Source: CAD feature listing. Evaluate the final solid. Frame: model axes, mm. A direction names the side the tool comes from. Round coordinates to 2 decimals unless told otherwise and drop trailing zeros. Loops run counter-clockwise (first coordinate to the right, second up) from the corner with the lowest first, then second, coordinate; pieces in that order, holes last. Notation, with made-up numbers: (-25, 79) -> (24, 79) arc R28 cw to (24, 99) -> close; hole circle Ø2 at (55.5, 74). An arc over 180 degrees is marked (long way). Write item = value, one per line.
from build123d import *

# Parameters (mm, degrees)
EXTRUDE_1_DEPTH              = 7
HOLE_WIZARD_M3_2_D           = 3.2
HOLE_WIZARD_M3_2_DEPTH       = 7
HOLE_WIZARD_M3_2_CBORE_D     = 6.2
HOLE_WIZARD_M3_2_CBORE_DEPTH = 1.3
HOLE_WIZARD_M3_2_TIP         = 0.96137699
CUT_EXTRUDE_1_DEPTH          = 2
EXTRUDE_START                = -3.5
EXTRUDE_3_DEPTH              = 1.5
FILLET_1_R                   = 2
CHAMFER_1_SIZE               = 0.5
CHAMFER_1_SIZE2              = 0.866025404
FILLET_2_R                   = 1
CHAMFER_2_SIZE               = 0.5
DELETE_START                 = 2
DELETE_FACE_1_DEPTH          = 3
DELETE_FACE_2_DEPTH          = 3
FILLET_3_R                   = 3.5
CHAMFER_3_SIZE               = 0.3


with BuildPart() as part:
    # 草图1 → 凸台-拉伸1 (new body)
    with BuildSketch(Plane(origin=(0, 0, 0), x_dir=(1, 0, 0), z_dir=(0, 1, 0))):
        Polygon((12.5, -5.17766953), (12.5, 5.17766953), (5.17766953, 12.5), (-5.17766953, 12.5), (-12.5, 5.17766953), (-12.5, -5.17766953), (-5.17766953, -12.5), (5.17766953, -12.5), align=None)
    extrude(amount=EXTRUDE_1_DEPTH)

    # M3 六角圆柱头螺钉的柱形沉头孔2
    with Locations(Plane.XZ):
        with Locations((-5.25, 0), (0, 5.25), (5.25, 0), (0, -5.25)):
            CounterBoreHole(HOLE_WIZARD_M3_2_D / 2, HOLE_WIZARD_M3_2_CBORE_D / 2, HOLE_WIZARD_M3_2_CBORE_DEPTH, depth=HOLE_WIZARD_M3_2_DEPTH)
            with Locations((0, 0, -(HOLE_WIZARD_M3_2_DEPTH + HOLE_WIZARD_M3_2_TIP / 2))):  # 118° drill point
                Cone(0, HOLE_WIZARD_M3_2_D / 2, HOLE_WIZARD_M3_2_TIP, mode=Mode.SUBTRACT)

    # 草图7 → 切除-拉伸1 (cut)
    with BuildSketch(Plane(origin=(0, 7, 0), x_dir=(1, 0, 0), z_dir=(0, 1, 0))):
        with BuildLine():
            Line((-1, 2), (1, 2))
            ThreePointArc((1, 2), (3, 0), (1, -2))
            Line((1, -2), (-1, -2))
            ThreePointArc((-1, -2), (-3, 0), (-1, 2))
        make_face()
    extrude(amount=-CUT_EXTRUDE_1_DEPTH, mode=Mode.SUBTRACT)

    # 草图8 → 凸台-拉伸3 (add, symmetric)
    with BuildSketch(Plane(origin=(0, 7, 0), x_dir=(1, 0, 0), z_dir=(0, 1, 0)).offset(EXTRUDE_START)):
        Polygon((5.798989873, 14), (-5.798989873, 14), (-14, 5.798989873), (-14, -5.798989873), (-5.798989873, -14), (5.798989873, -14), (14, -5.798989873), (14, 5.798989873), align=None)
        Polygon((12.5, 5.17766953), (5.17766953, 12.5), (-5.17766953, 12.5), (-12.5, 5.17766953), (-12.5, -5.17766953), (-5.17766953, -12.5), (5.17766953, -12.5), (12.5, -5.17766953), align=None, mode=Mode.SUBTRACT)
    extrude(amount=EXTRUDE_3_DEPTH, both=True)

    # 圆角1
    fillet_1_edges = [part.edges().sort_by_distance(p)[0] for p in [
        (5.17766953, 6, 12.5),
        (-5.17766953, 6, 12.5),
        (-12.5, 6, 5.17766953),
        (-12.5, 6, -5.17766953),
        (-5.17766953, 6, -12.5),
        (5.17766953, 6, -12.5),
        (12.5, 6, -5.17766953),
        (12.5, 6, 5.17766953),
        (5.17766953, 1, 12.5),
        (-5.17766953, 1, 12.5),
        (-12.5, 1, 5.17766953),
        (-12.5, 1, -5.17766953),
        (-5.17766953, 1, -12.5),
        (5.17766953, 1, -12.5),
        (12.5, 1, -5.17766953),
        (12.5, 1, 5.17766953),
        (14, 3.5, -5.798989873),
        (5.798989873, 3.5, -14),
        (-5.798989873, 3.5, -14),
        (-14, 3.5, -5.798989873),
        (-14, 3.5, 5.798989873),
        (-5.798989873, 3.5, 14),
        (5.798989873, 3.5, 14),
        (14, 3.5, 5.798989873),
    ]]
    fillet(fillet_1_edges, radius=FILLET_1_R)

    # 倒角1
    chamfer_1_edges = [part.edges().sort_by_distance(p)[0] for p in [
        (-3, 7, 0),
        (0, 7, 2),
        (3, 7, 0),
        (0, 7, -2),
    ]]
    chamfer_1_side = [part.faces().sort_by_distance(p)[0] for p in [
        (12.146446609, 7, 0),
    ]]
    chamfer(chamfer_1_edges, length=CHAMFER_1_SIZE, length2=CHAMFER_1_SIZE2, reference=chamfer_1_side[0])

    # 圆角2
    fillet_2_edges = [part.edges().sort_by_distance(p)[0] for p in [
        (9.899494937, 2, -9.899494937),
        (9.899494937, 5, -9.899494937),
        (14, 2, 0),
        (9.899494937, 2, 9.899494937),
        (0, 2, 14),
        (-9.899494937, 2, 9.899494937),
        (-14, 2, 0),
        (-9.899494937, 2, -9.899494937),
        (0, 2, -14),
        (-13.847759065, 2, -5.735929613),
        (5.735929613, 2, -13.847759065),
        (-5.735929613, 2, -13.847759065),
        (-13.847759065, 2, 5.735929613),
        (-5.735929613, 2, 13.847759065),
        (5.735929613, 2, 13.847759065),
        (13.847759065, 2, 5.735929613),
        (13.847759065, 2, -5.735929613),
        (14, 5, 0),
        (0, 5, -14),
        (-9.899494937, 5, -9.899494937),
        (-14, 5, 0),
        (-9.899494937, 5, 9.899494937),
        (0, 5, 14),
        (9.899494937, 5, 9.899494937),
        (-13.847759065, 5, -5.735929613),
        (5.735929613, 5, -13.847759065),
        (-5.735929613, 5, -13.847759065),
        (-13.847759065, 5, 5.735929613),
        (-5.735929613, 5, 13.847759065),
        (5.735929613, 5, 13.847759065),
        (13.847759065, 5, 5.735929613),
        (13.847759065, 5, -5.735929613),
    ]]
    fillet(fillet_2_edges, radius=FILLET_2_R)

    # 倒角2
    chamfer_2_edges = [part.edges().sort_by_distance(p)[0] for p in [
        (12.5, 0, 0),
        (8.838834765, 0, 8.838834765),
        (0, 0, 12.5),
        (-8.838834765, 0, 8.838834765),
        (-12.5, 0, 0),
        (-8.838834765, 0, -8.838834765),
        (0, 0, -12.5),
        (8.838834765, 0, -8.838834765),
        (-12.347759065, 0, -5.11460927),
        (12.347759065, 0, -5.11460927),
        (5.11460927, 0, -12.347759065),
        (-5.11460927, 0, -12.347759065),
        (-12.347759065, 0, 5.11460927),
        (-5.11460927, 0, 12.347759065),
        (5.11460927, 0, 12.347759065),
        (12.347759065, 0, 5.11460927),
        (0, 7, 12.5),
        (-8.838834765, 7, 8.838834765),
        (8.838834765, 7, 8.838834765),
        (12.5, 7, 0),
        (8.838834765, 7, -8.838834765),
        (0, 7, -12.5),
        (-8.838834765, 7, -8.838834765),
        (-12.5, 7, 0),
        (12.347759065, 7, 5.11460927),
        (5.11460927, 7, 12.347759065),
        (12.347759065, 7, -5.11460927),
        (5.11460927, 7, -12.347759065),
        (-5.11460927, 7, -12.347759065),
        (-12.347759065, 7, -5.11460927),
        (-12.347759065, 7, 5.11460927),
        (-5.11460927, 7, 12.347759065),
    ]]
    chamfer(chamfer_2_edges, length=CHAMFER_2_SIZE)

    # Delete Face 1: read off the stored shape, not the designer's step
    # Delete Face 1 outline → Delete Face 1 (add)
    with BuildSketch(Plane(origin=(0, 0, 0), x_dir=(1, 0, 0), z_dir=(0, 1, 0)).offset(DELETE_START)):
        with BuildLine():
            ThreePointArc((13.414213562, -6.384776311), (13.847759065, -5.735929613), (14, -4.970562748))
            Line((14, -4.970562748), (14, 4.970562748))
            ThreePointArc((14, 4.970562748), (13.847759065, 5.735929613), (13.414213562, 6.384776311))
            Line((13.414213562, 6.384776311), (6.384776311, 13.414213562))
            ThreePointArc((6.384776311, 13.414213562), (5.735929613, 13.847759065), (4.970562748, 14))
            Line((4.970562748, 14), (-4.970562748, 14))
            ThreePointArc((-4.970562748, 14), (-5.735929613, 13.847759065), (-6.384776311, 13.414213562))
            Line((-6.384776311, 13.414213562), (-13.414213562, 6.384776311))
            ThreePointArc((-13.414213562, 6.384776311), (-13.847759065, 5.735929613), (-14, 4.970562748))
            Line((-14, 4.970562748), (-14, -4.970562748))
            ThreePointArc((-14, -4.970562748), (-13.847759065, -5.735929613), (-13.414213562, -6.384776311))
            Line((-13.414213562, -6.384776311), (-6.384776311, -13.414213562))
            ThreePointArc((-6.384776311, -13.414213562), (-5.735929613, -13.847759065), (-4.970562748, -14))
            Line((-4.970562748, -14), (4.970562748, -14))
            ThreePointArc((4.970562748, -14), (5.735929613, -13.847759065), (6.384776311, -13.414213562))
            Line((6.384776311, -13.414213562), (13.414213562, -6.384776311))
        make_face()
        with BuildLine():
            ThreePointArc((4.349242405, 12.5), (5.11460927, 12.347759065), (5.763455967, 11.914213562))
            Line((5.763455967, 11.914213562), (11.914213562, 5.763455967))
            ThreePointArc((11.914213562, 5.763455967), (12.347759065, 5.11460927), (12.5, 4.349242405))
            Line((12.5, 4.349242405), (12.5, -4.349242405))
            ThreePointArc((12.5, -4.349242405), (12.347759065, -5.11460927), (11.914213562, -5.763455967))
            Line((11.914213562, -5.763455967), (5.763455967, -11.914213562))
            ThreePointArc((5.763455967, -11.914213562), (5.11460927, -12.347759065), (4.349242405, -12.5))
            Line((4.349242405, -12.5), (-4.349242405, -12.5))
            ThreePointArc((-4.349242405, -12.5), (-5.11460927, -12.347759065), (-5.763455967, -11.914213562))
            Line((-5.763455967, -11.914213562), (-11.914213562, -5.763455967))
            ThreePointArc((-11.914213562, -5.763455967), (-12.347759065, -5.11460927), (-12.5, -4.349242405))
            Line((-12.5, -4.349242405), (-12.5, 4.349242405))
            ThreePointArc((-12.5, 4.349242405), (-12.347759065, 5.11460927), (-11.914213562, 5.763455967))
            Line((-11.914213562, 5.763455967), (-5.763455967, 11.914213562))
            ThreePointArc((-5.763455967, 11.914213562), (-5.11460927, 12.347759065), (-4.349242405, 12.5))
            Line((-4.349242405, 12.5), (4.349242405, 12.5))
        make_face(mode=Mode.SUBTRACT)
    extrude(amount=DELETE_FACE_1_DEPTH)

    # Delete Face 2: read off the stored shape, not the designer's step
    # Delete Face 2 outline → Delete Face 2 (add)
    with BuildSketch(Plane(origin=(0, 0, 0), x_dir=(1, 0, 0), z_dir=(0, 1, 0)).offset(DELETE_START)):
        with BuildLine():
            Line((14, 5.798989873), (13.414213562, 6.384776311))
            ThreePointArc((13.414213562, 6.384776311), (13.847759065, 5.735929613), (14, 4.970562748))
            Line((14, 4.970562748), (14, 5.798989873))
        make_face()
        with BuildLine():
            ThreePointArc((4.970562748, 14), (5.735929613, 13.847759065), (6.384776311, 13.414213562))
            Line((6.384776311, 13.414213562), (5.798989873, 14))
            Line((5.798989873, 14), (4.970562748, 14))
        make_face()
        with BuildLine():
            Line((14, -5.798989873), (14, -4.970562748))
            ThreePointArc((14, -4.970562748), (13.847759065, -5.735929613), (13.414213562, -6.384776311))
            Line((13.414213562, -6.384776311), (14, -5.798989873))
        make_face()
        with BuildLine():
            ThreePointArc((-6.384776311, 13.414213562), (-5.735929613, 13.847759065), (-4.970562748, 14))
            Line((-4.970562748, 14), (-5.798989873, 14))
            Line((-5.798989873, 14), (-6.384776311, 13.414213562))
        make_face()
        with BuildLine():
            Line((5.798989873, -14), (6.384776311, -13.414213562))
            ThreePointArc((6.384776311, -13.414213562), (5.735929613, -13.847759065), (4.970562748, -14))
            Line((4.970562748, -14), (5.798989873, -14))
        make_face()
        with BuildLine():
            ThreePointArc((-14, 4.970562748), (-13.847759065, 5.735929613), (-13.414213562, 6.384776311))
            Line((-13.414213562, 6.384776311), (-14, 5.798989873))
            Line((-14, 5.798989873), (-14, 4.970562748))
        make_face()
        with BuildLine():
            Line((-5.798989873, -14), (-4.970562748, -14))
            ThreePointArc((-4.970562748, -14), (-5.735929613, -13.847759065), (-6.384776311, -13.414213562))
            Line((-6.384776311, -13.414213562), (-5.798989873, -14))
        make_face()
        with BuildLine():
            ThreePointArc((-13.414213562, -6.384776311), (-13.847759065, -5.735929613), (-14, -4.970562748))
            Line((-14, -4.970562748), (-14, -5.798989873))
            Line((-14, -5.798989873), (-13.414213562, -6.384776311))
        make_face()
    extrude(amount=DELETE_FACE_2_DEPTH)

    # 圆角3
    fillet_3_edges = [part.edges().sort_by_distance(p)[0] for p in [
        (14, 3.5, -5.798989873),
        (14, 3.5, 5.798989873),
        (5.798989873, 3.5, 14),
        (-5.798989873, 3.5, 14),
        (-14, 3.5, 5.798989873),
        (-14, 3.5, -5.798989873),
        (-5.798989873, 3.5, -14),
        (5.798989873, 3.5, -14),
    ]]
    fillet(fillet_3_edges, radius=FILLET_3_R)

    # 倒角3
    chamfer_3_edges = [part.edges().sort_by_distance(p)[0] for p in [
        (9.899494937, 2, 9.899494936),
        (9.899494937, 5, 9.899494936),
        (9.899494936, 2, -9.899494937),
        (14, 2, 0),
        (0, 2, 14),
        (-9.899494936, 2, 9.899494937),
        (-14, 2, 0),
        (-9.899494937, 2, -9.899494936),
        (0, 2, -14),
        (-5.688634418, 2, 13.733578364),
        (-13.733578364, 2, 5.688634418),
        (-13.733578364, 2, -5.688634418),
        (-5.688634418, 2, -13.733578364),
        (5.688634418, 2, -13.733578364),
        (13.733578364, 2, -5.688634418),
        (13.733578364, 2, 5.688634418),
        (5.688634418, 2, 13.733578364),
        (0, 5, 14),
        (14, 5, 0),
        (9.899494936, 5, -9.899494937),
        (0, 5, -14),
        (-9.899494937, 5, -9.899494936),
        (-14, 5, 0),
        (-9.899494936, 5, 9.899494937),
        (-5.688634418, 5, 13.733578364),
        (-13.733578364, 5, 5.688634418),
        (-13.733578364, 5, -5.688634418),
        (-5.688634418, 5, -13.733578364),
        (5.688634418, 5, -13.733578364),
        (13.733578364, 5, -5.688634418),
        (13.733578364, 5, 5.688634418),
        (5.688634418, 5, 13.733578364),
    ]]
    chamfer(chamfer_3_edges, length=CHAMFER_3_SIZE)


solid = part.part
1. Section query A-A (x = 0). Give the number of separate pieces and of enclosed holes in the cut face, then the cut area to 3 significant figures.
Evaluation:
separate_pieces = 3
enclosed_holes = 0
area = 122 mm²
2. Mould query, pull axis X, two halves, no side actions, for faces 4 (the face through (13.726, 3.517, -5.706)), 5 (the face through (0, 1, 12.5)), 6 (the face through (0, 5.6, 2)). Classes: released by +X, released by -X, zero draft, split by the parting line, or undercut.
Evaluation:
face_4 = released by +X
face_5 = zero draft
face_6 = undercut
3. Contact query for flat-ended pins moving along their axis: pin 1 Ø0.6 at (x, y) = (0.5, 5.5) entering from +Z; pin 2 Ø1.9 at (x, z) = (-4, -1) entering from -Y; pin 3 Ø1.2 at (y, z) = (1.5, 1) entering from +X; pin 4 Ø3 at (x, z) = (-0.5, -3.5) entering from -Y. Output: stop coordinate, or through.
Evaluation:
pin_1 = 12.5
pin_2 = 1.3
pin_3 = 13.8
pin_4 = 0
4. Set-up query: faces 1 (the face through (1.3, 1.3, 3.9)), 2 (the face through (5.125, 1.26, -12.344)), 3 (the face through (5.125, 5.76, -12.344)). Return all of +Z, -Z, +X, -X, +Y, -Y with unobstructed straight access to the full face (end or side cutting, diameter ignored); none if empty.
Evaluation:
face_1 = -Y
face_2 = -Z, +X, -Y
face_3 = -Z, +X, +Y
5. Section query D-D (z = 9.25). Return the cut outline in (x, y).
Evaluation:
outline = (-10.55, 2.3) -> (-10.12, 2) -> (-8.43, 2) -> (-8.43, 0.5) -> (-7.72, 0) -> (7.72, 0) -> (8.43, 0.5) -> (8.43, 2) -> (10.12, 2) -> (10.55, 2.3) -> (10.55, 4.7) -> (10.12, 5) -> (8.43, 5) -> (8.43, 6.5) -> (7.72, 7) -> (-7.72, 7) -> (-8.43, 6.5) -> (-8.43, 5) -> (-10.12, 5) -> (-10.55, 4.7) -> close
6. Section query B-B (y = 3.25). Return the cut outline in (x, z).
Evaluation:
outline = (-14, -4.35) arc R3.5 ccw to (-12.97, -6.82) -> (-6.82, -12.97) arc R3.5 ccw to (-4.35, -14) -> (4.35, -14) arc R3.5 ccw to (6.82, -12.97) -> (12.97, -6.82) arc R3.5 ccw to (14, -4.35) -> (14, 4.35) arc R3.5 ccw to (12.97, 6.82) -> (6.82, 12.97) arc R3.5 ccw to (4.35, 14) -> (-4.35, 14) arc R3.5 ccw to (-6.82, 12.97) -> (-12.97, 6.82) arc R3.5 ccw to (-14, 4.35) -> close; hole circle Ø3.2 at (-5.25, 0); hole circle Ø3.2 at (0, -5.25); hole circle Ø3.2 at (0, 5.25); hole circle Ø3.2 at (5.25, 0)
7. Line query: probe 1 along Z at (x, y) = (0, 0.7); probe 2 along Z at (x, y) = (0, 4.5). Output: solid intervals per line, ascending. Write a range as from..to.
Evaluation:
probe_1 = -12.5..-8.35, -2.15..2.15, 8.35..12.5
probe_2 = -14..-6.85, -3.65..3.65, 6.85..14
